Geometry: final body of the model. Coordinates: model frame, mm. A direction names the side the tool comes from. Give positions to 0.01 mm unless a question says otherwise; leave off trailing zeros. Answer in a Markdown table with one row per item.
from build123d import *

# Parameters (mm, degrees)
SKETCH1_W           = 150
SKETCH1_H           = 49
BOSS_EXTRUDE1_DEPTH = 39
CUT_EXTRUDE1_DEPTH  = 0.5
CUT_EXTRUDE2_DEPTH  = 0.5
FILLET1_R           = 4
FILLET2_R           = 1


with BuildPart() as part:
    # Sketch1 → Boss-Extrude1 (new body)
    with BuildSketch(Plane(origin=(0, 0, -15), x_dir=(-1, 0, 0), z_dir=(0, 0, -1))):
        with Locations((6, 2.5)):
            Rectangle(SKETCH1_W, SKETCH1_H)
    extrude(amount=-BOSS_EXTRUDE1_DEPTH)

    # Sketch2 → Cut-Extrude1 (cut)
    with BuildSketch(Plane(origin=(69, 0, 0), x_dir=(0, 0, -1), z_dir=(1, 0, 0))):
        with BuildLine():
            Line((-19.125, 12.875), (-19.125, -7.875))
            ThreePointArc((-19.125, -7.875), (-16.781854249, -13.531854249), (-11.125, -15.875))
            Line((-11.125, -15.875), (2.125, -15.875))
            ThreePointArc((2.125, -15.875), (7.781854249, -13.531854249), (10.125, -7.875))
            Line((10.125, -7.875), (10.125, 12.875))
            ThreePointArc((10.125, 12.875), (7.781854249, 18.531854249), (2.125, 20.875))
            Line((2.125, 20.875), (-11.125, 20.875))
            ThreePointArc((-11.125, 20.875), (-16.781854249, 18.531854249), (-19.125, 12.875))
        make_face()
    extrude(amount=-CUT_EXTRUDE1_DEPTH, mode=Mode.SUBTRACT)

    # Sketch3 → Cut-Extrude2 (cut)
    with BuildSketch(Plane.ZY.offset(81)):
        with BuildLine():
            Line((11.125, 20.875), (-2.125, 20.875))
            ThreePointArc((-2.125, 20.875), (-7.781854249, 18.531854249), (-10.125, 12.875))
            Line((-10.125, 12.875), (-10.125, -7.875))
            ThreePointArc((-10.125, -7.875), (-7.781854249, -13.531854249), (-2.125, -15.875))
            Line((-2.125, -15.875), (11.125, -15.875))
            ThreePointArc((11.125, -15.875), (16.781854249, -13.531854249), (19.125, -7.875))
            Line((19.125, -7.875), (19.125, 12.875))
            ThreePointArc((19.125, 12.875), (16.781854249, 18.531854249), (11.125, 20.875))
        make_face()
    extrude(amount=-CUT_EXTRUDE2_DEPTH, mode=Mode.SUBTRACT)

    # Fillet1
    fillet1_edges = [part.edges().sort_by_distance(p)[0] for p in [
        (-81, 2.5, 24),
        (69, 2.5, 24),
        (-81, 2.5, -15),
        (69, 2.5, -15),
    ]]
    fillet(fillet1_edges, radius=FILLET1_R)

    # Fillet2
    fillet2_edges = [part.edges().sort_by_distance(p)[0] for p in [
        (-6, -22, -15),
        (-6, 27, -15),
        (-81, 27, 4.5),
        (-6, 27, 24),
        (69, 27, 4.5),
        (67.828427125, 27, 22.828427125),
        (67.828427125, 27, -13.828427125),
        (-79.828427125, 27, 22.828427125),
        (-79.828427125, 27, -13.828427125),
        (-81, -22, 4.5),
        (69, -22, 4.5),
        (-6, -22, 24),
        (67.828427125, -22, 22.828427125),
        (67.828427125, -22, -13.828427125),
        (-79.828427125, -22, 22.828427125),
        (-79.828427125, -22, -13.828427125),
    ]]
    fillet(fillet2_edges, radius=FILLET2_R)


solid = part.part
Q1. Material intervals for line 1 along X through (y, z) = (-9.5, 1), sorted ascending.
Check values:
| item | result |
|---|---|
| line 1 | -80.5 to 68.5 |
Q2. First-contact query: pin 1 (8 mm diameter, centred on y = 9, z = -4.5, fed in from -X); pin 2 (9 mm diameter, centred on y = -2.5, z = 6.5, fed in from +X); pin 3 (0.6 mm diameter, centred on x = 69, z = 4, fed in from -Y). Flat tips, straight axial feed; report the tip coordinate or a pass-through.
Check values:
| item | result |
|---|---|
| pin 1 | x = -80.5 |
| pin 2 | x = 68.5 |
| pin 3 | y = -21.71 |
Q3. Reachability of faces 4 (the cylindrical face through (-80.754, -13.469, -7.844)), 5 (the cylindrical face through (68.754, -13.594, -7.719)), 6 (the flat face through (-5, -22, 4)) from +Z, -Z, +X, -X, +Y, -Y: full face, straight path, thin tool, end or side. Return the list, or none.
Check values:
| item | result |
|---|---|
| face 4 | -X |
| face 5 | +X |
| face 6 | +Z, -Z, +X, -X, -Y |
Q4. Draft query along Y for faces 1 (the flat face through (-5, 27, 4)), 2 (the flat face through (69, 0.6, -10.5)), 3 (the flat face through (-80.5, 3, 4)). Return one class per face: pulls with the +Y half, pulls with the -Y half, needs draft (parallel to the pull), parting line crosses it, or undercut.
Check values:
| item | result |
|---|---|
| face 1 | pulls with the +Y half |
| face 2 | needs draft |
| face 3 | undercut |
